Verification items for the finished model (mm, model axes). A direction names the side the tool comes from. Give positions to 0.01 mm unless a question says otherwise; leave off trailing zeros. Order: outer loops, then holes, each group sorted by start corner. A loop starts at its lowest first (then second) coordinate and runs counter-clockwise, first axis right, second up.
from build123d import *

# Parameters (mm, degrees)
SKICA1_R                = 1.75
P_IDAT_VYSUNUT_M1_DEPTH = 3


with BuildPart() as part:
    # Skica1 → Přidat vysunutím1 (new body)
    with BuildSketch(Plane.XY):
        Polygon((20, 3), (35, 3), (35, 0), (55, 0), (55, 3), (70, 3), (70, 0), (77.5, 0), (77.5, 11), (77.5, 20.346281592), (77.5, 41.653718408), (77.5, 51), (77.5, 62), (70, 62), (70, 59), (55, 59), (55, 62), (35, 62), (35, 59), (20, 59), (20, 62), (0, 62), (0, 0), (20, 0), align=None)
        with Locations((41.5, 47)):
            Circle(SKICA1_R, mode=Mode.SUBTRACT)
        with Locations(Location((41.5, 15, 0), (0, 0, 180))):
            Circle(SKICA1_R, mode=Mode.SUBTRACT)
        with Locations((73.5, 15)):
            Circle(SKICA1_R, mode=Mode.SUBTRACT)
        with Locations(Location((73.5, 47, 0), (0, 0, 180))):
            Circle(SKICA1_R, mode=Mode.SUBTRACT)
        Polygon((65.5, 51), (49.5, 51), (37.5, 39), (37.5, 23), (49.5, 11), (65.5, 11), (76.500000683, 22.000000683), (76.500000683, 39.999999317), align=None, mode=Mode.SUBTRACT)
    p_idat_vysunut_m1 = extrude(amount=P_IDAT_VYSUNUT_M1_DEPTH)

    # Zrcadlit1: Přidat vysunutím1 across plane
    add(p_idat_vysunut_m1.mirror(Plane(origin=(77.5, 51, 3), x_dir=(0, 0, 1), z_dir=(-1, 0, 0))))


solid = part.part
(1) Release check for a two-part mould opening along Y. For faces 1 (the flat face through (63, 59, 1)), 2 (the flat face through (83.9, 45.4, 1.5)), 3 (the flat face through (79, 45, 0)) record: pulls with the +Y half, pulls with the -Y half, needs draft (parallel to the pull), parting line crosses it, or undercut.
Solved:
face 1: pulls with the +Y half
face 2: undercut
face 3: needs draft
(2) Section check A-A, the plane x = 53. Enter the section's corners in (y, z), then the cut area to 3 significant figures.
Solved:
outline: (0, 0) - (11, 0) - (11, 3) - (0, 3) - close; (51, 0) - (62, 0) - (62, 3) - (51, 3) - close
area: 66.0 mm2
(3) Section check C-C, the plane y = 15. Enter the section's corners in (x, z).
Solved:
outline: (0, 0) - (39.75, 0) - (39.75, 3) - (0, 3) - close; (43.25, 0) - (45.5, 0) - (45.5, 3) - (43.25, 3) - close; (69.5, 0) - (71.75, 0) - (71.75, 3) - (69.5, 3) - close; (75.25, 0) - (79.75, 0) - (79.75, 3) - (75.25, 3) - close; (83.25, 0) - (85.5, 0) - (85.5, 3) - (83.25, 3) - close; (109.5, 0) - (111.75, 0) - (111.75, 3) - (109.5, 3) - close; (115.25, 0) - (155, 0) - (155, 3) - (115.25, 3) - close
(4) Go/stop test with flat-tipped pins: pin 1 (0.9 mm diameter, centred on x = 95, z = 2, fed in from -Y); pin 2 (3 mm diameter, centred on x = 41.5, y = 47, fed in from +Z). Record where each tip stops, or that it passes through.
Solved:
pin 1: stops at y = 3
pin 2: passes through
(5) Section check D-D, the plane x = 113.5. Enter the section's corners in (y, z), then the cut area to 3 significant figures.
Solved:
outline: (0, 0) - (13.25, 0) - (13.25, 3) - (0, 3) - close; (16.75, 0) - (19, 0) - (19, 3) - (16.75, 3) - close; (43, 0) - (45.25, 0) - (45.25, 3) - (43, 3) - close; (48.75, 0) - (62, 0) - (62, 3) - (48.75, 3) - close
area: 93.0 mm2
(6) Set-up check for faces 4 (the flat face through (135, 60, 1)), 5 (the flat face through (84.1, 16.4, 1.5)), 6 (the flat face through (120, 2, 1)): record each of +Z, -Z, +X, -X, +Y, -Y from which the full face is reachable in a straight line by a thin tool's end or side.
Solved:
face 4: +Z, -Z, +Y
face 5: +Z, -Z
face 6: +Z, -Z, -Y
(7) Section check B-B, the plane y = 33. Enter the section's corners in (x, z), then the cut area to 3 significant figures.
Solved:
outline: (0, 0) - (37.5, 0) - (37.5, 3) - (0, 3) - close; (76.5, 0) - (78.5, 0) - (78.5, 3) - (76.5, 3) - close; (117.5, 0) - (155, 0) - (155, 3) - (117.5, 3) - close
area: 231 mm2
(8) Scan lines: line 1 (X direction, y = 30, z = 2.1); line 2 (Y direction, x = 91, z = 1.6); line 3 (Y direction, x = 41.5, z = 1.7). Record each from-to range of solid material in increasing order.
Solved:
line 1: x = 0 to 37.5, 76.5 to 78.5, 117.5 to 155
line 2: y = 3 to 11, 51 to 59
line 3: y = 0 to 13.25, 16.75 to 19, 43 to 45.25, 48.75 to 62
